The listing builds one solid part. Answer for the finished solid, in the listing's coordinates (mm). Face numbers are marked on the shaded views. A direction names the side the tool comes from. Round coordinates to 2 decimals unless told otherwise and drop trailing zeros. Order: outer loops, then holes, each group sorted by start corner. A loop starts at its lowest first (then second) coordinate and runs counter-clockwise, first axis right, second up. Notation, with made-up numbers: (-1.75, 55.25) - (24.25, 55.25) arc R15 ccw to (24.25, 66.25) - close; hole circle Ø2 at (52.5, 2.5). An arc over 180 degrees is marked (long way). One line per item, written item: value. Start each with the question number.
1. Section B-B, the plane x = -9 is taken. Give the vertices of the cut face in (y, z).
2. Straight lines are drawn through the part: line 1 (X direction, y = -5.5, z = -19) (3 decimals); line 2 (X direction, y = -21.5, z = 22) (3 decimals); line 3 (Z direction, x = 26, y = -19.25). For each, find the intervals that lie inside material, in ascending order.
3. Section A-A, the plane z = -18.5 is taken. Give the vertices of the cut face in (x, y) (3 decimals), then the cut area to 3 significant figures.
4. A tool of negligible diameter and unlimited length cuts with its end or side. For the marked faces 1 and 2, from which of +Z, -Z, +X, -X, +Y, -Y can it reach the whole face along a straight path? Write none if from no direction.
5. For a pull along X with two mould halves and no side action, classify the marked faces 3, 4 and 5 as released by +X, released by -X, zero draft, split by the parting line, or undercut.
6. Section C-C, the plane y = -4.75 is taken. Give the vertices of the cut face in (x, z) (3 decimals), then the cut area to 3 significant figures.
7. A flat-ended cylindrical pin translates along its axis: P1, Ø10, axis at x = -1, z = 19, coming from the +Y side (1 decimal). Find the tip coordinate at first contact, or state that the pin passes through.
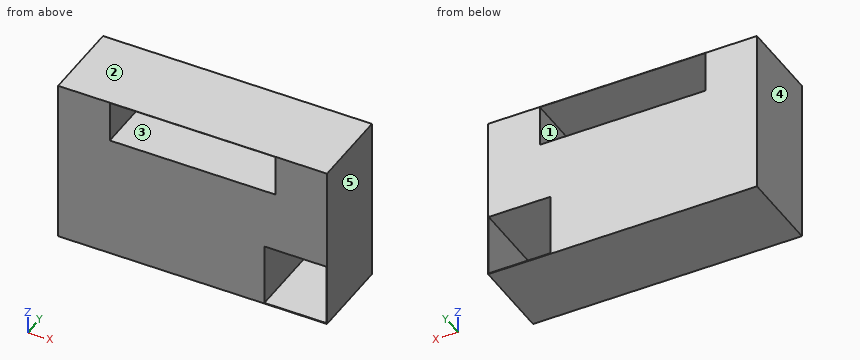
from build123d import *

# Parameters (mm, degrees)
F0_W     = 82.55
F0_H     = 50.8
F1_DEPTH = 25.4
F2_W     = 50.8
F2_H     = 12.7
F3_DEPTH = 50.292
F4_W     = 19.05
F4_H     = 19.05
F5_DEPTH = 72.644


with BuildPart() as f1:
    # F0 (on Front) → F1 (new body)
    with BuildSketch(Plane.XZ):
        Rectangle(F0_W, F0_H)
    extrude(amount=F1_DEPTH)

    # F2 (on Front) → F3 (cut)
    with BuildSketch(Plane.XZ):
        with Locations((0, 18.983158)):
            Rectangle(F2_W, F2_H)
    extrude(amount=F3_DEPTH, mode=Mode.SUBTRACT)

    # F4 (on Front) → F5 (cut)
    with BuildSketch(Plane.XZ):
        with Locations((31.582892, -15.641052)):
            Rectangle(F4_W, F4_H)
    extrude(amount=F5_DEPTH, mode=Mode.SUBTRACT)


solid = f1.part
Answer list:
1. outline: (-25.4, -25.4) - (0, -25.4) - (0, 12.63) - (-25.4, 12.63) - close; (-25.4, 25.33) - (0, 25.33) - (0, 25.4) - (-25.4, 25.4) - close
2. line 1: x = -41.275 to 22.058, 41.108 to 41.275
2. line 2: x = -41.275 to -25.4, 25.4 to 41.275
2. line 3: z = -25.4 to -25.17, -6.12 to 25.4
3. outline: (-41.275, -25.4) - (22.058, -25.4) - (22.058, 0) - (-41.275, 0) - close; (41.108, -25.4) - (41.275, -25.4) - (41.275, 0) - (41.108, 0) - close
3. area: 1,610 mm²
4. face 1: +Y, -Y
4. face 2: +Z, +X, -X, +Y, -Y
5. face 3: undercut
5. face 4: released by -X
5. face 5: released by +X
6. outline: (-41.275, -25.4) - (41.275, -25.4) - (41.275, 25.4) - (-41.275, 25.4) - close; hole (-25.4, 12.633) - (25.4, 12.633) - (25.4, 25.333) - (-25.4, 25.333) - close; hole (22.058, -25.166) - (41.108, -25.166) - (41.108, -6.116) - (22.058, -6.116) - close
6. area: 3,190 mm²
7. P1: passes through
